Design review of the part built by this model. Coordinates are the model's own, in mm. Face numbers are marked on the shaded views. A direction names the side the tool comes from. Coordinates: 2 decimals unless noted, no trailing zeros. Write each loop counter-clockwise with the first axis right and the second up, starting at its lowest first coordinate (ties: lowest second). Pieces come first, ordered by that corner, then holes.
Q1. Take a section at B-B (x = 18). Give the boundary of the cut face in (y, z).
Q2. Machinability: for the marked faces 1, 2, 3, 4 and 5, which of the approach directions +Z, -Z, +X, -X, +Y, -Y give a long, thin tool a straight path to every point of the face, cutting with its end or side? Answer none if there is none.
Q3. Insertion check: pin 1 (4 mm diameter, centred on x = 8, y = 4, fed in from -Z); pin 2 (2.5 mm diameter, centred on x = -7, y = -1, fed in from -Z); pin 3 (4 mm diameter, centred on x = 12, y = -2.5, fed in from +Z). Each pin has a flat end and moves straight along its axis. Give the tip position at first contact, or say it passes through.
Q4. For probe 1 along X at (y, z) = (-3.5, -2.25); probe 2 along Z at (x, y) = (26, 0); probe 3 along Y at (x, z) = (0.5, 1), list the stretches that pass through material, from the lowest coordinate up.
Q5. Take a section at A-A (y = 0). Give the boundary of the cut face in (x, z).
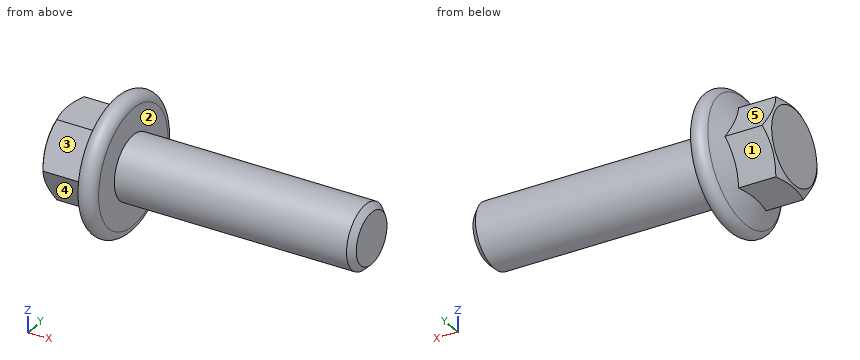
Autodesk Inventor part; units mm, degrees
ref_plane "Work Plane1" through (10.95, 0, 0) normal (0, 0, -1) x (1, 0, 0)
ref_plane "YZ Plane" through (0, 0, 0) normal (1, 0, 0) x (0, 1, 0)
ref_plane "XZ Plane" through (0, 0, 0) normal (0, 1, 0) x (-1, 0, 0)
sketch "Sketch1" plane through (0, 0, 0) normal (0, 0, 1) x (1, 0, 0)
  line L0 (-3.825, 0) -> (-3.825, 4.5101)
  line L1 (0, 7.3) -> (0, 4)
  line L2 (8, 4) -> (30, 4)
  line L3 (30, 4) -> (30, 0)
  line L4 (30, 0) -> (-3.825, 0)
  arc A0 (0, 7.3) -> (-2.2876, 7.8071) centre (-1.2, 7.3) ccw
  line L5 (0, -1.745) -> (0, 10.4702)
  line L6 (-11.59, 0) -> (42.765, 0)
  line L7 (0, 4) -> (0.0001, 4)
  line L8 (0.0001, 4) -> (0.0001, 4)
  line L9 (0.0001, 4) -> (7.2332, 4)
  line L10 (7.2332, 4) -> (8, 4)
  line L11 (-3.825, 4.5101) -> (-2.2876, 7.8071)
  line L12 (0.0001, 4) -> (8, 4) construction
  line L13 (8, 4) -> (8, 0) construction
  dimension "d0" = 1.2
  dimension "d1" = 30
  dimension "d2" = 22
  dimension "d3" = 17
  dimension "d4" = 8
  dimension "d5" = 3.825
  dimension "d15" = 8
  dimension "d16" = 8
  dimension "d17" = 0.0001
  dimension "d18" = 0.7668
  dimension "d19" = 25
revolve "Body" add sketch "Sketch1" angle 360 about axis through (30, 0, 0) along (-1, 0, 0)
sketch "Sketch2" plane through (0, 0, 0) normal (1, 0, 0) x (0, 0, -1)
  line L0 (5, 2.8868) -> (5, -2.8868)
  line L1 (5, -2.8868) -> (0, -5.7735)
  line L2 (0, -5.7735) -> (-5, -2.8868)
  line L3 (-5, -2.8868) -> (-5, 2.8868)
  line L4 (-5, 2.8868) -> (0, 5.7735)
  line L5 (0, 5.7735) -> (5, 2.8868)
  point P0 (0, 0)
  point P1 (0, 0)
  dimension "d23" = 10
extrude "Head" add sketch "Sketch2" against normal blind 8.5
sketch "Sketch3" plane through (0, 0, 0) normal (0, 0, 1) x (1, 0, 0)
  line L0 (-8.5, 4.75) -> (-8.5, 5.7735)
  line L1 (-8.5, 5.7735) -> (-7.9091, 5.7735)
  line L2 (-7.9091, 5.7735) -> (-8.5, 4.75)
  line L3 (-9.5528, 0) -> (-2.183, 0)
  line L4 (-8.5, 5.7735) -> (-8.5, 2.8868)
  line L5 (-3.2359, 5.7735) -> (-8.5, 5.7735)
  point P0 (-8.5, 2.8868)
  dimension "d8" = 30
  dimension "d22" = 9.5
revolve "Chamfer1" cut sketch "Sketch3" angle 360 about axis through (-10, 0, 0) along (1, 0, 0)
thread "Thread"
chamfer "Chamfer2" distance 0.7668 distance2 0.7668 1 edges at (30, -4, 0) measured on face at (30, 0.9825, 0.2422)
ref_plane "Work Plane1" through (10.95, 0, 0) normal (0, 0, -1) x (1, 0, 0)
equation "\"d0\" = PHH"
equation "\"d1\" = NLG"
equation "\"d2\" = GEL"
equation "\"d3\" = LADI"
equation "\"d4\" = GD"
equation "\"d5\" = 0.45 * KOH"
equation "\"d15\" = SD2"
equation "\"d16\" = BDM"
equation "\"d18\" = GAL"
equation "\"d19\" = KEWI"
equation "\"d23\" = SW"
equation "\"d6\" = KOH"
equation "\"d8\" = ANG1"
equation "\"d22\" = SW0"
equation "\"d10\" = GEL"
equation "\"d13\" = -0.5 * SPD + 0.5 * GD"
equation "\"d14\" = GUL"
equation "\"NLG\" = 30"
equation "\"GD\" = NND"
equation "\"BDM\" = NND"
equation "\"KOH\" = 8.5"
equation "\"GEL\" = 22"
equation "\"LADI\" = 17"
equation "\"SW\" = 10"
equation "\"PHH\" = RR"
equation "\"SW0\" = 9.5"
equation "\"SPD\" = NND - 1.2269 * PTC"
equation "\"SD2\" = NND"
equation "\"SD\" = 0"
equation "\"ANG1\" = 30deg"
equation "\"KEWI\" = 25deg"
equation "\"GAL\" = 0.61345 * PTC"
equation "\"GUL\" = 0.61345 * PTC"
equation "\"PTC\" = 1.25"
equation "\"THREADDIA\" = 8"
equation "\"E0\" = 1.155 * SW"
equation "\"TOA\" = 30deg"
equation "\"NND\" = 8"
equation "\"GD1\" = THREADDIA - 1.2269 * PTC"
equation "\"KOH1\" = 3.8"
equation "\"RR\" = 1.2"
properties part number "PWTR-0134" material "Stainless Steel"
Response:
1. outline: circle Ø8 at (0, 0)
2. face 1: -Z, -X, +Y
2. face 2: +X
2. face 3: +Z, -X, -Y
2. face 4: -Z, -X, -Y
2. face 5: +Z, -X, +Y
3. pin 1: stops at z = -3.46
3. pin 2: stops at z = -5
3. pin 3: stops at z = 3.97
4. probe 1: x = -8.5 to 0
4. probe 2: z = -4 to 4
4. probe 3: y = -3.87 to 3.87
5. outline: (-8.5, -4.75) - (-8.36, -5) - (-3.6, -5) - (-2.29, -7.81) arc R1.2 ccw to (0, -7.3) - (0, -4) - (29.23, -4) - (30, -3.23) - (30, 3.23) - (29.23, 4) - (0, 4) - (0, 7.3) arc R1.2 ccw to (-2.29, 7.81) - (-3.6, 5) - (-8.36, 5) - (-8.5, 4.75) - close
